```python
from build123d import *

# Parameters (mm, degrees)
BOSS_EXTRU_1_DEPTH = 1


with BuildPart() as part:
    # Esquisse1 → Boss.-Extru.1 (new body)
    with BuildSketch(Plane.XY):
        with BuildLine():
            Line((12, 11.7), (13.5, 11.7))
            Line((13.5, 11.7), (13.5, 14.7))
            Line((13.5, 14.7), (15, 14.7))
            ThreePointArc((15, 14.7), (19.25, 18.95), (15, 23.2))
            Line((15, 23.2), (-3, 23.2))
            ThreePointArc((-3, 23.2), (-7.25, 18.95), (-3, 14.7))
            Line((-3, 14.7), (-1.5, 14.7))
            Line((-1.5, 14.7), (-1.5, 11.7))
            Line((-1.5, 11.7), (0, 11.7))
            Line((0, 11.7), (0, 0))
            Line((0, 0), (12, 0))
            Line((12, 0), (12, 11.7))
        make_face()
        with BuildLine():
            Line((15, 20.1), (13.5, 20.1))
            Line((13.5, 20.1), (13.5, 17.8))
            Line((13.5, 17.8), (15, 17.8))
            ThreePointArc((15, 17.8), (16.15, 18.95), (15, 20.1))
        make_face(mode=Mode.SUBTRACT)
        with BuildLine():
            Line((-3, 20.1), (-1.5, 20.1))
            Line((-1.5, 20.1), (-1.5, 17.8))
            Line((-1.5, 17.8), (-3, 17.8))
            ThreePointArc((-3, 17.8), (-4.15, 18.95), (-3, 20.1))
        make_face(mode=Mode.SUBTRACT)
    extrude(amount=BOSS_EXTRU_1_DEPTH)


solid = part.part
```
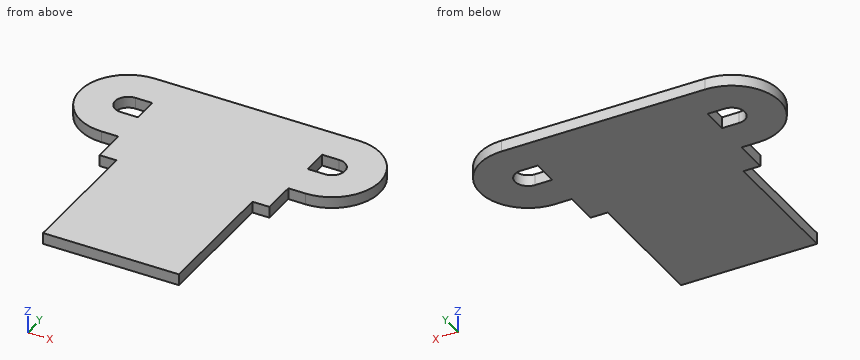
Check sheet for the modelled part. Datum: model origin and axes. Units: mm. Give positions to 0.01 mm unless a question says otherwise; leave off trailing zeros. Write each loop counter-clockwise with the first axis right and the second up, starting at its lowest first coordinate (ties: lowest second). Pieces come first, ordered by that corner, then holes. Notation, with made-up numbers: (-16.75, -20) - (23.25, -20) arc R31 cw to (23.25, 18) - close; hole circle Ø8 at (2, 51). An arc over 180 degrees is marked (long way). Answer as a JSON object with one key per item and string values. Group by question number.
1) Sectioned sample at C-C (z = 0.35). Record the cut outline in (x, y), then the cut area to 3 significant figures.
2) Sectioned sample at B-B (x = -2). Record the cut outline in (y, z), then the cut area to 3 significant figures.
3) Sectioned sample at D-D (y = 5). Record the cut outline in (x, z).
4) Thickness scan on probe 1 along X at (y, z) = (19, 0.5); probe 2 along X at (y, z) = (8.75, 0.1); probe 3 along Y at (x, z) = (-3.5, 0.8). Record the ranges inside material, lowest first. Write a range as from..to.
5) Depth check by flat-ended pin: P1, Ø0.5, axis at x = -2, z = 0.5, coming from the -Y side. Enter the tip coordinate at first touch or a pass-through.
6) Sectioned sample at A-A (y = 18.95). Record the cut outline in (x, z).
Geometry results:
{
 "1": {"outline": "(-3, 14.7) - (-1.5, 14.7) - (-1.5, 11.7) - (0, 11.7) - (0, 0) - (12, 0) - (12, 11.7) - (13.5, 11.7) - (13.5, 14.7) - (15, 14.7) arc R4.25 ccw to (15, 23.2) - (-3, 23.2) arc R4.25 ccw to start; hole (-3, 17.8) - (-1.5, 17.8) - (-1.5, 20.1) - (-3, 20.1) arc R1.15 ccw to start; hole (13.5, 17.8) - (15, 17.8) arc R1.15 ccw to (15, 20.1) - (13.5, 20.1) - close", "area": "384 mm^2"},
 "2": {"outline": "(14.7, 0) - (17.8, 0) - (17.8, 1) - (14.7, 1) - close; (20.1, 0) - (23.2, 0) - (23.2, 1) - (20.1, 1) - close", "area": "6.20 mm^2"},
 "3": {"outline": "(0, 0) - (12, 0) - (12, 1) - (0, 1) - close"},
 "4": {"probe 1": "x = -7.25..-4.15, -1.5..13.5, 16.15..19.25", "probe 2": "x = 0..12", "probe 3": "y = 14.73..17.91, 19.99..23.17"},
 "5": {"P1": "stops at y = 14.7"},
 "6": {"outline": "(-7.25, 0) - (-4.15, 0) - (-4.15, 1) - (-7.25, 1) - close; (-1.5, 0) - (13.5, 0) - (13.5, 1) - (-1.5, 1) - close; (16.15, 0) - (19.25, 0) - (19.25, 1) - (16.15, 1) - close"}
}
